Autodesk Inventor part; units mm, degrees
ref_plane "YZ Plane" through (0, 0, 0) normal (1, 0, 0) x (0, 1, 0)
ref_plane "XZ Plane" through (0, 0, 0) normal (0, 1, 0) x (-1, 0, 0)
ref_plane "XY Plane" through (0, 0, 0) normal (0, 0, 1) x (1, 0, 0)
sketch "Sketch1" plane through (0, 0, 0) normal (0, 0, 1) x (1, 0, 0)
  circle A0 centre (0, 0) radius 3.175
  line L0 (3.2079, 5.5563) -> (6.4158, 0)
  line L1 (6.4158, 0) -> (3.2079, -5.5562)
  line L2 (3.2079, -5.5562) -> (-3.2079, -5.5562)
  line L3 (-3.2079, -5.5562) -> (-6.4158, 0)
  line L4 (-6.4158, 0) -> (-3.2079, 5.5563)
  line L5 (-3.2079, 5.5563) -> (3.2079, 5.5563)
  dimension "d0" = 6.35
  dimension "d1" = 11.1125
extrude "Extrusion1" add sketch "Sketch1" against normal blind 25.4 contours A0
extrude "Extrusion2" add sketch "Sketch1" along normal blind 3.175 contours A0 | L0 L1 L2 L3 L4 L5
thread "Thread1"
chamfer "Chamfer1" distance 0.7937 angle 45 6 edges at (4.8119, 2.7781, 3.175) (0, 5.5563, 3.175) (-4.8119, 2.7781, 3.175) (-4.8119, -2.7781, 3.175) (0, -5.5562, 3.175) (4.8119, -2.7781, 3.175)
properties part number "1_bolt_.25_20"
Build history of the part. All positions in model axes, mm. A direction names the side the tool comes from. Give positions to 0.01 mm unless a question says otherwise; leave off trailing zeros. Loops run counter-clockwise (first coordinate to the right, second up) from the corner with the lowest first, then second, coordinate; pieces in that order, holes last. Notation, with made-up numbers: (27.25, 33.5) -> (48.25, 33.5) arc R7 ccw to (48.25, 39.5) -> close; hole circle Ø6 at (-40, 71.25). An arc over 180 degrees is marked (long way). One line per question, with ' | ' between items.
Q1. Tool access for faces 1 (the cylindrical face through (-0.69, -3.1, -12.52)), 2 (the flat face through (-4.44, 2.62, 2.78)): list every direction of +Z, -Z, +X, -X, +Y, -Y with a clear straight run to the whole face (end or side of a thin tool).
Filled sheet:
face 1: -Z | face 2: +Z, -X, +Y
Q2. Cut at A-A, the plane x = 0. Write the cut outline in (y, z) (1 decimal).
Filled sheet:
outline: (-5.6, 0) -> (-3.2, 0) -> (-3.2, -25.4) -> (3.2, -25.4) -> (3.2, 0) -> (5.6, 0) -> (5.6, 2.4) -> (4.8, 3.2) -> (-4.8, 3.2) -> (-5.6, 2.4) -> close
Q3. Drop flat-ended pins along their axis: pin 1 (5 mm diameter, centred on x = -3, z = -17.5, fed in from +Y); pin 2 (6 mm diameter, centred on x = -3.5, z = -2, fed in from -Y); pin 3 (5 mm diameter, centred on x = 1, z = -20.5, fed in from -Y) (3 decimals); pin 4 (3 mm diameter, centred on x = 2.5, z = -11.5, fed in from +Y). Give the stop position or say it passes through.
Filled sheet:
pin 1: stops at y = 3.14 | pin 2: stops at y = -5.56 | pin 3: stops at y = -3.175 | pin 4: stops at y = 3.01
Q4. Drill centre lines: line 1 along Z through (x, y) = (1, -3.5) (3 decimals); line 2 along X through (y, z) = (1, -12.5); line 3 along X through (y, z) = (-2.75, -17.25). Where is each one in solid material? Low to high. Write a range as [from, to].
Filled sheet:
line 1: z = [0, 3.175] | line 2: x = [-3.01, 3.01] | line 3: x = [-1.59, 1.59]
Q5. Cut at B-B, the plane y = 1. Write the cut outline in (x, z) (3 decimals).
Filled sheet:
outline: (-5.838, 0) -> (-3.013, 0) -> (-3.013, -25.4) -> (3.013, -25.4) -> (3.013, 0) -> (5.838, 0) -> (5.838, 2.381) -> (4.922, 3.175) -> (-4.922, 3.175) -> (-5.838, 2.381) -> close
Q6. Cut at D-D, the plane y = 3.75. Write the cut outline in (x, z) (3 decimals).
Filled sheet:
outline: (-4.251, 0) -> (4.251, 0) -> (4.251, 2.381) -> (3.334, 3.175) -> (-3.334, 3.175) -> (-4.251, 2.381) -> close
Q7. Cut at C-C, the plane z = -20.5. Write the cut outline in (x, y) (3 decimals).
Filled sheet:
outline: circle Ø6.35 at (0, 0)
